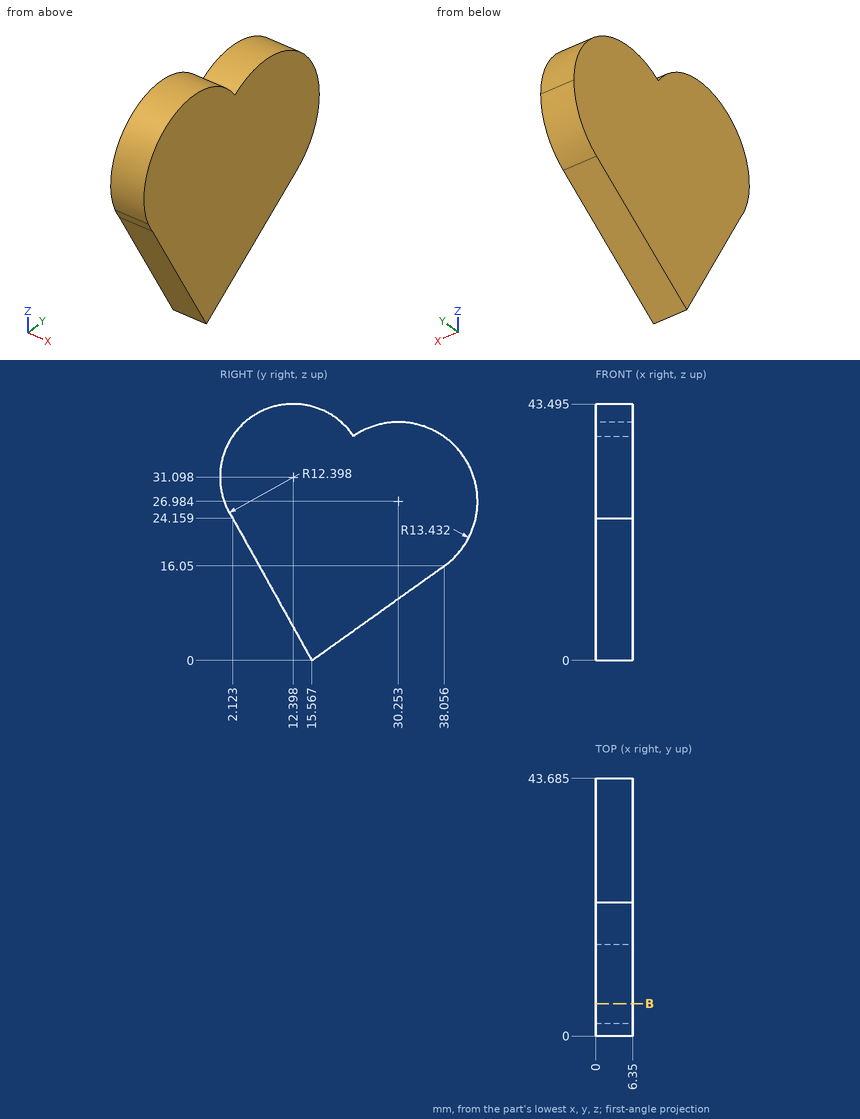
Answer from the drawing. Dimensions are ordinates in mm from the lowest x, y and z of the part. Round coordinates to 2 decimals unless told otherwise and drop trailing zeros. Loops run counter-clockwise (first coordinate to the right, second up) from the corner with the lowest first, then second, coordinate; pieces in that order, holes last.
1) A cutting plane is placed at B-B on y = 5.5. Determine the outline of the cut face in (x, z).
Outcome:
outline: (0, 18.09) - (6.35, 18.09) - (6.35, 41.4) - (0, 41.4) - close
2) Given P1, Ø2, axis at x = 1, z = 22.5, coming from the -Y side; P2, Ø6, axis at y = 16, z = 31.5, coming from the -X side; P3, Ø1, axis at x = 1.5, z = 8, coming from the +Y side (1 decimal); P4, Ø3, axis at x = 1.5, z = 35.5, coming from the +Y side, each flat-ended and moving along its own axis, determine where each tip first touches the part or whether it passes through.
Outcome:
P1: stops at y = 2.49
P2: stops at x = 0
P3: stops at y = 27.5
P4: stops at y = 41.71
3) Consider line 1 (Y direction, x = 2.75, z = 4); line 2 (Y direction, x = 5.5, z = 30); line 3 (Z direction, x = 3.25, y = 28.5). Determine where each line is inside the solid, lowest interval first.
Outcome:
line 1: y = 13.34 to 21.17
line 2: y = 0.05 to 43.34
line 3: z = 9.23 to 40.3
